Solid Edge part; units mm, degrees
sketch "Sketch1" plane through (0, 0, 0) normal (0, 0, 1) x (1, 0, 0)
  line L0 (-9.5, -13) -> (9.5, -13)
  line L1 (9.5, -13) -> (9.5, 13)
  line L2 (9.5, 13) -> (-9.5, 13)
  line L3 (-9.5, 13) -> (-9.5, -13)
  dimension "D1" = 9.5
  dimension "D2" = 9.5
extrude "Ajout_matière_1" add sketch "Sketch1" along normal blind 17.5
fillet "Congé_1" radius 1 12 edges at (9.5, 0, 17.5) (-9.5, 0, 17.5) (-9.5, 0, 0) (9.5, 0, 0) (0, -13, 0) (-9.5, -13, 8.75) (0, -13, 17.5) (9.5, -13, 8.75) (0, 13, 17.5) (-9.5, 13, 8.75) (0, 13, 0) (9.5, 13, 8.75)
sketch "Sketch2" plane through (0, 13, 8.75) normal (0, 1, 0) x (0, 0, -1)
  circle A0 centre (0, 0) radius 1.5
extrude "Ajout_matière_2" add sketch "Sketch2" along normal blind 18
cosmetic_thread "Thread1"
properties material "Acier S235"
Geometry check sheet. Reference: the model listing, model coordinates, mm. A direction names the side the tool comes from. Round coordinates to 2 decimals unless told otherwise and drop trailing zeros. Loops run counter-clockwise (first coordinate to the right, second up) from the corner with the lowest first, then second, coordinate; pieces in that order, holes last. Notation, with made-up numbers: (14, 61.5) - (27, 61.5) arc R18 ccw to (27, 68.5) - close; hole circle Ø8 at (64.25, 79). An arc over 180 degrees is marked (long way). Write item = value, one per line. Start each with the question number.
1. Section check A-A on z = 2.25. Enter the section's corners in (x, y).
2. Depth check by flat-ended pin: pin 1 (5 mm diameter, centred on x = -1.5, z = 2.5, fed in from +Y); pin 2 (10 mm diameter, centred on y = 19, z = 10.5, fed in from +X). Enter the tip coordinate at first touch or a pass-through.
3. Section check D-D on y = 18. Enter the section's corners in (x, z), then the cut area to 3 significant figures.
4. Section check B-B on x = 0. Enter the section's corners in (y, z), then the cut area to 3 significant figures.
5. Thickness scan on line 1 (Y direction, x = -3.5, z = 8.5); line 2 (X direction, y = -5.5, z = 0.5); line 3 (Z direction, x = 7.25, y = 12.5). Record the ranges inside material, lowest first.
6. Set-up check for faces 1 (the face through (0.07, 21.87, 10.25)), 2 (the face through (-9.5, 0, 9)): record each of +Z, -Z, +X, -X, +Y, -Y from which the full face is reachable in a straight line by a thin tool's end or side.
7. Section check C-C on z = 8.75. Enter the section's corners in (x, y), then the cut area to 3 significant figures.
Working result:
q1.outline = (-9.5, -12) arc R1 ccw to (-8.5, -13) - (8.5, -13) arc R1 ccw to (9.5, -12) - (9.5, 12) arc R1 ccw to (8.5, 13) - (-8.5, 13) arc R1 ccw to (-9.5, 12) - close
q2.pin_1 = 13
q2.pin_2 = 1.5
q3.outline = circle Ø3 at (0, 8.75)
q3.area = 7.07 mm^2
q4.outline = (-13, 1) arc R1 ccw to (-12, 0) - (12, 0) arc R1 ccw to (13, 1) - (13, 7.25) - (31, 7.25) - (31, 10.25) - (13, 10.25) - (13, 16.5) arc R1 ccw to (12, 17.5) - (-12, 17.5) arc R1 ccw to (-13, 16.5) - close
q4.area = 508 mm^2
q5.line_1 = -13 to 13
q5.line_2 = -9.37 to 9.37
q5.line_3 = 0.13 to 17.37
q6.face_1 = +Y
q6.face_2 = +Z, -Z, -X, +Y, -Y
q7.outline = (-9.5, -12) arc R1 ccw to (-8.5, -13) - (8.5, -13) arc R1 ccw to (9.5, -12) - (9.5, 12) arc R1 ccw to (8.5, 13) - (1.5, 13) - (1.5, 31) - (-1.5, 31) - (-1.5, 13) - (-8.5, 13) arc R1 ccw to (-9.5, 12) - close
q7.area = 547 mm^2
